Check sheet for the modelled part. Datum: model origin and axes. Units: mm. A direction names the side the tool comes from. Coordinates: 2 decimals unless noted, no trailing zeros. Loops run counter-clockwise (first coordinate to the right, second up) from the corner with the lowest first, then second, coordinate; pieces in that order, holes last. Notation, with made-up numbers: (-1.75, -13) - (48.25, -13) arc R36 cw to (48.25, 22) - close; hole circle Ø8 at (-29, -27). An arc over 180 degrees is marked (long way). Use a Markdown table: item, result. Add a question column.
1) Thickness scan on line 1 (Y direction, x = -0.7, z = -12.5); line 2 (Y direction, x = 12, z = 0.75); line 3 (Z direction, x = 20, y = 7). Record the ranges inside material, lowest first.
2) Sectioned sample at C-C, the plane x = 11.25. Enter the section's corners in (y, z).
3) Sectioned sample at B-B, the plane z = -14.5. Enter the section's corners in (x, y).
4) Draft check along Y on faces 1 (the cylindrical face through (-0.76, 29.487, -12.695)), 2 (the flat face through (11, 20, 1.5)). Enter one of: pulls with the +Y half, pulls with the -Y half, needs draft (parallel to the pull), parting line crosses it, or undercut.
5) Go/stop test with flat-tipped pins: P1, Ø1.8, axis at y = 28, z = -12.5, coming from the +X side; P2, Ø3, axis at y = 10, z = -15, coming from the +X side; P3, Ø4.5, axis at x = 12, y = 3, coming from the -Z side. Record where each tip stops, or that it passes through.
6) Sectioned sample at D-D, the plane y = 28. Enter the section's corners in (x, z), then the cut area to 4 significant figures.
7) Tool access check on faces 3 (the flat face through (24, 20, 1)), 4 (the flat face through (0, 15, -12)). Record the directions out of +Z, -Z, +X, -X, +Y, -Y that give a thin tool (end or side, any length) a straight path to the whole face; none if there is none.
8) Sectioned sample at A-A, the plane y = 37. Enter the section's corners in (x, z), then the cut area to 4 significant figures.
from build123d import *

# Parameters (mm, degrees)
BOSS_EXTRUDE1_DEPTH = 40
SKETCH3_R           = 3.9
SKETCH3_R_2         = 1.5
CUT_EXTRUDE1_DEPTH  = 1.5
SKETCH4_R           = 1.7
CUT_EXTRUDE2_DEPTH  = 10


with BuildPart() as part:
    # Sketch2 → Boss-Extrude1 (new body)
    with BuildSketch(Plane(origin=(0, 0, 0), x_dir=(1, 0, 0), z_dir=(0, 1, 0))):
        Polygon((0, 0), (0, 24), (-1.5, 24), (-1.5, -1.5), (24, -1.5), (24, 0), align=None)
    extrude(amount=BOSS_EXTRUDE1_DEPTH)

    # Sketch3 → Cut-Extrude1 (cut)
    with BuildSketch(Plane.ZY.offset(1.5)):
        with Locations((-12.5, 20)):
            Circle(SKETCH3_R)
        with Locations((-12.5, 28)):
            Circle(SKETCH3_R_2)
        with Locations((-12.5, 12)):
            Circle(SKETCH3_R_2)
    extrude(amount=-CUT_EXTRUDE1_DEPTH, mode=Mode.SUBTRACT)

    # Sketch4 → Cut-Extrude2 (cut)
    with BuildSketch(Plane(origin=(0, 0, 0), x_dir=(-1, 0, 0), z_dir=(0, 0, -1))):
        with Locations((-12, 3)):
            Circle(SKETCH4_R)
        with Locations((-12, 37)):
            Circle(SKETCH4_R)
    extrude(amount=-CUT_EXTRUDE2_DEPTH, mode=Mode.SUBTRACT)


solid = part.part
Solved:
| question | item | result |
|---|---|---|
| 1 | line 1 | y = 0 to 10.5, 13.5 to 16.1, 23.9 to 26.5, 29.5 to 40 |
| 1 | line 2 | y = 0 to 1.3, 4.7 to 35.3, 38.7 to 40 |
| 1 | line 3 | z = 0 to 1.5 |
| 2 | outline | (0, 0) - (1.47, 0) - (1.47, 1.5) - (0, 1.5) - close; (4.53, 0) - (35.47, 0) - (35.47, 1.5) - (4.53, 1.5) - close; (38.53, 0) - (40, 0) - (40, 1.5) - (38.53, 1.5) - close |
| 3 | outline | (-1.5, 0) - (0, 0) - (0, 16.65) - (-1.5, 16.65) - close; (-1.5, 23.35) - (0, 23.35) - (0, 40) - (-1.5, 40) - close |
| 4 | face 1 | undercut |
| 4 | face 2 | needs draft |
| 5 | P1 | passes through |
| 5 | P2 | stops at x = 0 |
| 5 | P3 | stops at z = 0 |
| 6 | outline | (-1.5, -24) - (0, -24) - (0, -14) - (-1.5, -14) - close; (-1.5, -11) - (0, -11) - (0, 0) - (24, 0) - (24, 1.5) - (-1.5, 1.5) - close |
| 6 | area | 69.75 mm2 |
| 7 | face 3 | +Z, -Z, +X, +Y, -Y |
| 7 | face 4 | -Z, +X, +Y, -Y |
| 8 | outline | (-1.5, -24) - (0, -24) - (0, 0) - (10.3, 0) - (10.3, 1.5) - (-1.5, 1.5) - close; (13.7, 0) - (24, 0) - (24, 1.5) - (13.7, 1.5) - close |
| 8 | area | 69.15 mm2 |
